Autodesk Inventor part; units mm, degrees
ref_plane "YZ Plane" through (0, 0, 0) normal (1, 0, 0) x (0, 1, 0)
ref_plane "XZ Plane" through (0, 0, 0) normal (0, 1, 0) x (-1, 0, 0)
ref_plane "XY Plane" through (0, 0, 0) normal (0, 0, 1) x (1, 0, 0)
sketch "Sketch1" plane through (0, 0, 0) normal (0, 1, 0) x (-1, 0, 0)
  circle A0 centre (0, 0) radius 6.35
  dimension "d0" = 12.7
extrude "Extrusion1" add sketch "Sketch1" along normal blind 146
sketch "Sketch3" plane through (0, 146, 0) normal (0, 1, 0) x (1, 0, 0)
  point P0 (0, 0)
  point P1 (0, 0)
hole "Hole2" at (0, 146, 0) direction (0, -1, 0) diameter 6 depth 10 tip angle 118
thread "Thread3"
sketch "Sketch4" plane through (0, 0, 0) normal (0, -1, 0) x (1, 0, 0)
  circle A0 centre (0, 0) radius 6.35
hole "Hole3" at (0, 0, 0) direction (0, 1, 0) diameter 6 depth 10 tip angle 118
thread "Thread4"
properties part number "Poste"
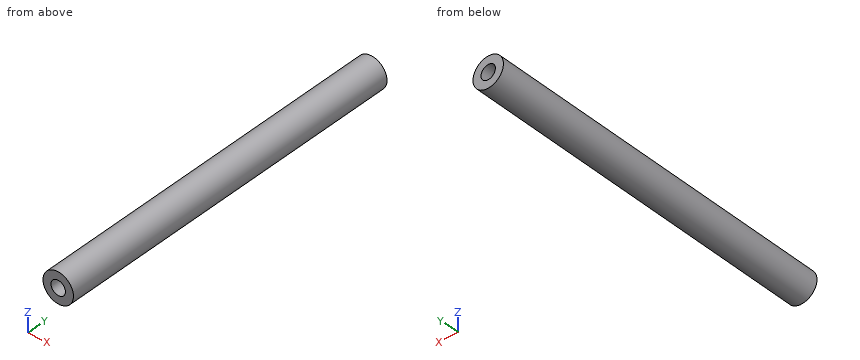
Check sheet for the modelled part. Datum: model origin and axes. Units: mm. Round coordinates to 2 decimals unless told otherwise and drop trailing zeros. Loops run counter-clockwise (first coordinate to the right, second up) from the corner with the lowest first, then second, coordinate; pieces in that order, holes last.
1. Scan lines: probe 1 along Z at (x, y) = (0, 139.25); probe 2 along X at (y, z) = (76, 0.5); probe 3 along X at (y, z) = (10, 0.5). Record each from-to range of solid material in increasing order.
2. Gauge pin test, flat ends, axial feed: pin 1 Ø2 at (x, z) = (-4, 4.5) entering from -Y; pin 2 Ø5.5 at (x, z) = (0, 0) entering from -Y; pin 3 Ø1.5 at (x, z) = (-1, 0.5) entering from -Y. Record the tip position at first contact, or that the pin passes through.
3. Sectioned sample at B-B on x = -4.5. Record the boundary of the cut face in (y, z), and give its area (3 significant figures).
4. Sectioned sample at A-A on y = 55. Record the boundary of the cut face in (x, z).
Recorded:
1. probe 1: z = -6.35 to -3, 3 to 6.35
1. probe 2: x = -6.33 to 6.33
1. probe 3: x = -6.33 to -2.96, 2.96 to 6.33
2. pin 1: stops at y = 0
2. pin 2: stops at y = 10.15
2. pin 3: stops at y = 10.68
3. outline: (0, -4.48) - (146, -4.48) - (146, 4.48) - (0, 4.48) - close
3. area: 1,310 mm2
4. outline: circle Ø12.7 at (0, 0)
